Can you work these out from the model? Positions are in its coordinate system, mm. A direction names the side the tool comes from. Coordinates: 2 decimals unless noted, no trailing zeros. Write each loop counter-clockwise with the first axis right and the second up, starting at its lowest first coordinate (ties: lowest second). Pieces come first, ordered by that corner, then holes. Notation, with made-up numbers: (-0.75, 35) - (5.25, 35) arc R16 ccw to (5.25, 52) - close; hole circle Ø1 at (17, -9). An arc over 180 degrees is marked (long way). One line per question, with ' | ' between items. Start each with the question number.
from build123d import *

# Parameters (mm, degrees)
BOSS_EXTRUDE1_DEPTH = 116
SKETCH2_W           = 118
SKETCH2_H           = 161
BOSS_EXTRUDE2_DEPTH = 2
SKETCH3_W           = 161
SKETCH3_H           = 167
BOSS_EXTRUDE4_DEPTH = 2


with BuildPart() as part:
    # Sketch1 → Boss-Extrude1 (new body)
    with BuildSketch(Plane.XY):
        Polygon((0, 0), (87.5, 0), (0, 134.5), align=None)
    extrude(amount=BOSS_EXTRUDE1_DEPTH)

    # Sketch2 → Boss-Extrude2 (add)
    with BuildSketch(Plane(origin=(0, 0, 0), x_dir=(-1, 0, 0), z_dir=(0, -1, 0))):
        with Locations((-59, -58)):
            Rectangle(SKETCH2_W, SKETCH2_H)
    extrude(amount=BOSS_EXTRUDE2_DEPTH)

    # Sketch3 → Boss-Extrude4 (add)
    with BuildSketch(Plane.ZY):
        with Locations((58, 81.5)):
            Rectangle(SKETCH3_W, SKETCH3_H)
    extrude(amount=BOSS_EXTRUDE4_DEPTH)


solid = part.part
(1) If we section it at B-B on x = 31.5: List the corners of the cut face in (y, z) for me, plus the area to 3 significant figures.
(2) If I drill on probe 1 along X at (y, z) = (81.5, -9); probe 2 along Z at (x, y) = (47.5, 19), over which ranges is the centre line in solid material (lowest first)?
(3) I'm going to push flat-ended pins straight in: pin 1 (4 mm diameter, centred on x = 62, z = 92.5, fed in from +Y); pin 2 (5 mm diameter, centred on x = 34, z = 32.5, fed in from +Y); pin 3 (10 mm diameter, centred on y = 71, z = 47.5, fed in from +X). Where does each tip first touch, or does it pass through?
(4) Which directions (+Z, -Z, +X, -X, +Y, -Y) give clear straight access to the entire face, cutting with the end or side of a thin tool? Please do faces 1 (the face through (24, 38, 116)), 2 (the face through (24, 38, 0)), 3 (the face through (0, 139, 57)), 4 (the face through (59, -2, 57)).
(5) If we section it at C-C on y = 112.5: List the corners of the cut face in (x, z) for me.
(6) If we section it at D-D on z = -3: List the corners of the cut face in (x, y) for me.
(7) If we section it at A-A on z = 60: List the corners of the cut face in (x, y) for me.
Values:
1) outline: (-2, -22.5) - (0, -22.5) - (0, 0) - (86.08, 0) - (86.08, 116) - (0, 116) - (0, 138.5) - (-2, 138.5) - close | area: 10,300 mm2
2) probe 1: -2 to 0 | probe 2: 0 to 116
3) pin 1: y = 42.27 | pin 2: y = 86.08 | pin 3: x = 44.56
4) face 1: +Z, +X, +Y | face 2: -Z, +X, +Y | face 3: +X, +Y | face 4: +Z, -Z, +X, -X, -Y
5) outline: (-2, -22.5) - (0, -22.5) - (0, 0) - (14.31, 0) - (14.31, 116) - (0, 116) - (0, 138.5) - (-2, 138.5) - close
6) outline: (-2, -2) - (118, -2) - (118, 0) - (0, 0) - (0, 165) - (-2, 165) - close
7) outline: (-2, -2) - (118, -2) - (118, 0) - (87.5, 0) - (0, 134.5) - (0, 165) - (-2, 165) - close
